from build123d import *

# Parameters (mm, degrees)
EXTRUDE_1_DEPTH            = 1
SKETCH_3_W                 = 0.814720046
SKETCH_3_H                 = 0.814720046
CUT_EXTRUDE_1_DEPTH        = 3.5
CHAMFER_1_SIZE             = 0.25
CHAMFER_1_OF_MIRROR_1_SIZE = 0.25
EXTRUDE_2_DEPTH            = 0.25
CHAMFER_2_SIZE             = 0.1
CHAMFER_2_SIZE2            = 0.4
CUT_EXTRUDE_2_DEPTH        = 8.514818694


with BuildPart() as part:
    # 草图1 → 凸台-拉伸1 (new, symmetric)
    with BuildSketch(Plane(origin=(0, 0, 0), x_dir=(0, 0, -1), z_dir=(1, 0, 0))):
        Polygon((-2.25, 0), (2.25, 0), (2.25, -4.3), (1.75, -4.3), (1.75, -3.8), (-1.75, -3.8), (-1.75, -4.3), (-2.25, -4.3), align=None)
    extrude(amount=EXTRUDE_1_DEPTH, both=True)

    # 草图3 → 切除-拉伸1 (cut)
    with BuildSketch(Plane(origin=(0, 0, 0), x_dir=(1, 0, 0), z_dir=(0, 1, 0))):
        with Locations((0, 1)):
            Rectangle(SKETCH_3_W, SKETCH_3_H)
    cut_extrude_1 = extrude(amount=-CUT_EXTRUDE_1_DEPTH, mode=Mode.SUBTRACT)

    # 倒角1
    chamfer_1_edges = [part.edges().sort_by_distance(p)[0] for p in [
        (-0.407360023, 0, -1),
        (0, 0, -0.592639977),
        (0.407360023, 0, -1),
        (0, 0, -1.407360023),
    ]]
    chamfer(chamfer_1_edges, length=CHAMFER_1_SIZE)

    # 镜向1: 切除-拉伸1 across plane
    add(cut_extrude_1.mirror(Plane.XY), mode=Mode.SUBTRACT)

    # 倒角1 of 镜向1
    chamfer_1_of_mirror_1_edges = [part.edges().sort_by_distance(p)[0] for p in [
        (-0.407360023, 0, 1),
        (0, 0, 0.592639977),
        (0.407360023, 0, 1),
        (0, 0, 1.407360023),
    ]]
    chamfer(chamfer_1_of_mirror_1_edges, length=CHAMFER_1_OF_MIRROR_1_SIZE)

    # 草图4 → 凸台-拉伸2 (add)
    with BuildSketch(Plane(origin=(0, 0, 0), x_dir=(0, 0, -1), z_dir=(1, 0, 0))):
        Polygon((1.562968954, -3.8), (1.1, -4.088782437), (1.1, -7.1), (0.9, -7.1), (0.9, -3.977816442), (1.18507098, -3.8), align=None)
    extrude(amount=EXTRUDE_2_DEPTH)

    # 倒角2
    chamfer_2_edges = [part.edges().sort_by_distance(p)[0] for p in [
        (0.25, -7.1, -1),
    ]]
    chamfer_2_side = [part.faces().sort_by_distance(p)[0] for p in [
        (0.125, -7.1, -1),
    ]]
    chamfer(chamfer_2_edges, length=CHAMFER_2_SIZE, length2=CHAMFER_2_SIZE2, reference=chamfer_2_side[0])

    # 草图5 → 切除-拉伸2 (cut, through all)
    with BuildSketch(Plane(origin=(0, 0, 0), x_dir=(1, 0, 0), z_dir=(0, 1, 0))):
        Polygon((0, 2.25), (-1, 2.25), (-1, -2.25), (1, -2.25), (1, 0), (0, 0), align=None)
    extrude(amount=-CUT_EXTRUDE_2_DEPTH, mode=Mode.SUBTRACT)

    # 镜向3: part across plane


with BuildPart() as part_1:
    add(part.part)
    add(part.part.mirror(Plane(origin=(0, 0, 0), x_dir=(0, 0, 1), z_dir=(1, 0, 0))))

    # 镜向4: part across plane


with BuildPart() as part_2:
    add(part_1.part)
    add(part_1.part.mirror(Plane(origin=(0, -7.1, 0), x_dir=(1, 0, 0), z_dir=(0, 0, -1))))


solid = part_2.part
CAD build for the part. Positions are in the model's coordinates, mm. A direction names the side the tool comes from. Give positions to 0.01 mm unless a question says otherwise; leave off trailing zeros. Order: outer loops, then holes, each group sorted by start corner. A loop starts at its lowest first (then second) coordinate and runs counter-clockwise, first axis right, second up. Notation, with made-up numbers: (60.5, 79) - (74.5, 79) arc R15 ccw to (74.5, 85) - close; hole circle Ø10 at (-31.75, 21). An arc over 180 degrees is marked (long way). Write each question's results on one line, items separated by ' | '.
1. Probe L1, parallel to Z at x = -0.25, y = -0.5; L2, parallel to X at y = -1.75, z = -0.8; L3, parallel to Z at x = -0.2, y = -6.5. List the from-to ranges inside material, lowest first. Write a range as from..to.
Calculated:
L1: z = -2.25..-1.41, -0.59..0.59, 1.41..2.25 | L2: x = -1..-0.41, 0.41..1 | L3: z = -1.1..-0.9, 0.9..1.1
2. Saw through at D-D on z = 1.9. List the corners of the cut face in (x, y), and give its area (3 significant figures).
Calculated:
outline: (-1, -4.3) - (1, -4.3) - (1, 0) - (-1, 0) - close | area: 8.60 mm2
3. Pin check, flat tips, straight feed: pin 1 (0.5 mm diameter, centred on y = -4.5, z = 1.5, fed in from +X); pin 2 (0.5 mm diameter, centred on y = -5, z = -1, fed in from -X). Stop position of each tip, or through.
Calculated:
pin 1: passes through | pin 2: stops at x = -0.25
4. Saw through at B-B on x = 0.8. List the corners of the cut face in (y, z), and give its area (3 significant figures).
Calculated:
outline: (-4.3, -2.25) - (0, -2.25) - (0, 2.25) - (-4.3, 2.25) - (-4.3, 1.75) - (-3.8, 1.75) - (-3.8, -1.75) - (-4.3, -1.75) - close | area: 17.6 mm2
5. 3-axis set-ups, long thin cutter, end or side, ignore diameter. For faces 4 (the face through (0, -2, -2.25)), 5 (the face through (0.407, -2, -1)): which of +Z, -Z, +X, -X, +Y, -Y reach the whole face in a straight line?
Calculated:
face 4: -Z, +X, -X, +Y, -Y | face 5: +Y
6. Pull direction Z, two halves, no side cores. Call faces 1 (the face through (0, -2, 2.25)), 2 (the face through (-0.407, -2, 1)), 3 (the face through (-1, -2, 0)): released by +Z, released by -Z, zero draft, split by the parting line, or undercut.
Calculated:
face 1: released by +Z | face 2: undercut | face 3: zero draft
7. Saw through at A-A on y = -4.5. List the corners of the cut face in (x, z), and give its area (3 significant figures).
Calculated:
outline: (-0.25, -1.1) - (0.25, -1.1) - (0.25, -0.9) - (-0.25, -0.9) - close; (-0.25, 0.9) - (0.25, 0.9) - (0.25, 1.1) - (-0.25, 1.1) - close | area: 0.200 mm2
8. Saw through at C-C on y = -1.25. List the corners of the cut face in (x, z), and give its area (3 significant figures).
Calculated:
outline: (-1, -2.25) - (1, -2.25) - (1, 2.25) - (-1, 2.25) - close; hole (-0.41, -1.41) - (0.41, -1.41) - (0.41, -0.59) - (-0.41, -0.59) - close; hole (-0.41, 0.59) - (0.41, 0.59) - (0.41, 1.41) - (-0.41, 1.41) - close | area: 7.67 mm2
